Part model, mm, in its own coordinate system. A direction names the side the tool comes from. Round coordinates to 2 decimals unless told otherwise and drop trailing zeros. Write each loop counter-clockwise with the first axis right and the second up, starting at its lowest first coordinate (ties: lowest second). Pieces come first, ordered by that corner, then holes. Notation, with made-up numbers: (58.5, -12.5) -> (86.5, -12.5) arc R25 ccw to (86.5, 7.5) -> close; hole circle Ø2 at (-5.5, 29.5). An arc over 180 degrees is marked (long way). Return JSON: item names as keys, results as strings. Group by question number.
```python
from build123d import *

# Parameters (mm, degrees)
BOX003_W     = 1000
BOX003_H     = 800
BOX003_DEPTH = 700
SKETCH_W     = 2000
SKETCH_H     = 1500
PAD_DEPTH    = 300


with BuildPart() as cube003:
    # Box003 → Box003 (new body)
    with BuildSketch(Plane(origin=(-122, -202, -351), x_dir=(1, 0, 0), z_dir=(0, 0, 1))):
        with Locations((500, 400)):
            Rectangle(BOX003_W, BOX003_H)
    extrude(amount=BOX003_DEPTH)


with BuildPart() as cut:
    # Sketch → Pad (new body)
    with BuildSketch(Plane.XZ):
        with Locations((-300, 0)):
            Rectangle(SKETCH_W, SKETCH_H)
    extrude(amount=PAD_DEPTH)

    # Cut: cut Cube003
    add(cube003.part, mode=Mode.SUBTRACT)


solid = cut.part
```
Item 1: Cut at C-C (z = 279.5). Write the cut outline in (x, y), then the cut area to 3 significant figures.
Item 2: Cut at A-A (y = -142). Write the cut outline in (x, z).
Item 3: Flat gauge pins, fed straight in: P1, Ø2, axis at y = -109, z = -71, coming from the +X side; P2, Ø8, axis at x = -993, z = 280.5, coming from the +Y side. Where does each tip first touch, or does it go through?
Item 4: Which spindle directions (+Z, -Z, +X, -X, +Y, -Y) get a long thin tool onto all of the face, cutting with end or side? Do faces 1 (the face through (283, -202, -6)), 2 (the face through (-314, -300, 10)). Say none if no direction does.
Item 5: Cut at B-B (x = 154.5). Write the cut outline in (y, z), then the cut area to 3 significant figures.
Item 6: Two-plate mould, pull along Z, no slides. Class faces 3 (the face through (-314, -148, -750)), 4 (the face through (-1300, -148, -10)), 5 (the face through (283, -100, -351)): released by +Z, released by -Z, zero draft, split by the parting line, or undercut.
Item 7: Wall check: L1, parallel to Z at x = -116, y = -40; L2, parallel to Y at x = -81, z = -327; L3, parallel to X at y = -132, z = 9.5. Give the ranges that are in metal, low to high.
Checks:
{
 "1": {"outline": "(-1300, -300) -> (700, -300) -> (700, -202) -> (-122, -202) -> (-122, 0) -> (-1300, 0) -> close", "area": "434,000 mm2"},
 "2": {"outline": "(-1300, -750) -> (700, -750) -> (700, -351) -> (-122, -351) -> (-122, 349) -> (700, 349) -> (700, 750) -> (-1300, 750) -> close"},
 "3": {"P1": "stops at x = -122", "P2": "stops at y = 0"},
 "4": {"face 1": "+X, +Y", "face 2": "+Z, -Z, +X, -X, -Y"},
 "5": {"outline": "(-300, -750) -> (0, -750) -> (0, -351) -> (-202, -351) -> (-202, 349) -> (0, 349) -> (0, 750) -> (-300, 750) -> close", "area": "309,000 mm2"},
 "6": {"face 3": "released by -Z", "face 4": "zero draft", "face 5": "undercut"},
 "7": {"L1": "z = -750 to -351, 349 to 750", "L2": "y = -300 to -202", "L3": "x = -1300 to -122"}
}
